For this review, take the finished solid that the model builds, in its own axes (mm). A direction names the side the tool comes from. Coordinates: 2 decimals unless noted, no trailing zeros. Loops run counter-clockwise (first coordinate to the right, second up) from the corner with the lowest first, then second, coordinate; pieces in that order, holes last. Notation, with made-up numbers: M 9.25,-27.75 L 28.25,-27.75 A18 cw 28.25,-14.75 Z; hole C 21,-25.75 d8. An arc over 180 degrees is marked long. Use one line per item in the form item = value.
```python
from build123d import *

# Parameters (mm, degrees)
BOSS_EXTRUDE1_DEPTH = 100
FILLET1_R           = 0.5
FILLET2_R           = 1


with BuildPart() as part:
    # Sketch1 → Boss-Extrude1 (new body)
    with BuildSketch(Plane.XY):
        Polygon((0, 0), (0, 12.7), (1.5875, 12.7), (1.5875, 1.5875), (12.7, 1.5875), (12.7, 0), align=None)
    extrude(amount=BOSS_EXTRUDE1_DEPTH)

    # Fillet1
    fillet1_edges = [part.edges().sort_by_distance(p)[0] for p in [
        (0, 0, 50),
    ]]
    fillet(fillet1_edges, radius=FILLET1_R)

    # Fillet2
    fillet2_edges = [part.edges().sort_by_distance(p)[0] for p in [
        (1.5875, 12.7, 50),
        (1.5875, 1.5875, 50),
        (12.7, 1.5875, 50),
    ]]
    fillet(fillet2_edges, radius=FILLET2_R)


solid = part.part
```
1. Consider section A-A on z = 11. Write out the cut boundary in (x, y), plus the area to 3 significant figures.
Computed values:
outline = M 0,0.5 A0.5 ccw 0.5,0 L 12.7,0 L 12.7,0.59 A1 ccw 11.7,1.59 L 2.59,1.59 A1 cw 1.59,2.59 L 1.59,11.7 A1 ccw 0.59,12.7 L 0,12.7 Z
area = 37.5 mm2
2. For pin 1 Ø7.5 at (x, z) = (9, 61) entering from +Y; pin 2 Ø4.5 at (y, z) = (7.5, 51.5) entering from +X, all flat-tipped, find the tip position at first contact; note any pin that passes through.
Computed values:
pin_1 = 1.59
pin_2 = 1.59
3. Consider section B-B on x = 8. Write out the cut boundary in (y, z), plus the area to 3 significant figures.
Computed values:
outline = M 0,0 L 1.59,0 L 1.59,100 L 0,100 Z
area = 159 mm2
4. Tool access review of faces 1 (the face through (7, 0, 49)), 2 (the face through (7, 1.588, 49)): name each direction out of +Z, -Z, +X, -X, +Y, -Y from which nothing blocks a thin tool from reaching the whole face with its end or side.
Computed values:
face_1 = +Z, -Z, +X, -X, -Y
face_2 = +Z, -Z, +X, +Y
5. Wall thickness on line 1 along Y through (x, z) = (9.5, 61); line 2 along X through (y, z) = (1.25, 73): over which ranges is each line inside the solid? List them lowest first. Write a range as from..to.
Computed values:
line_1 = 0..1.59
line_2 = 0..12.45
